Input: part model. Units: mm. Frame: model coordinates. Round coordinates to 2 decimals unless told otherwise and drop trailing zeros. Loops run counter-clockwise (first coordinate to the right, second up) from the corner with the lowest first, then second, coordinate; pieces in that order, holes last. Notation, with made-up numbers: (2, -32) -> (44, -32) arc R22 ccw to (44, -25) -> close; hole circle Ø3 at (87.25, -16.75). An arc over 180 degrees is marked (long way). Answer as a JSON object with one key per item and string values.
```python
from build123d import *

# Parameters (mm, degrees)
CYLINDER007_R     = 1.75
CYLINDER007_DEPTH = 5
CYLINDER006_R     = 1.75
CYLINDER006_DEPTH = 5
CYLINDER005_R     = 1.75
CYLINDER005_DEPTH = 5
CYLINDER004_R     = 1.75
CYLINDER004_DEPTH = 5
CUBE002_W         = 85
CUBE002_H         = 27
CUBE002_DEPTH     = 17
CYLINDER011_R     = 1.75
CYLINDER011_DEPTH = 5
CYLINDER010_R     = 1.75
CYLINDER010_DEPTH = 5
CYLINDER009_R     = 1.75
CYLINDER009_DEPTH = 5
CYLINDER008_R     = 1.75
CYLINDER008_DEPTH = 5
CUBE003_W         = 95.25
CUBE003_H         = 50.8
CUBE003_DEPTH     = 20.32
CYLINDER015_R     = 1.75
CYLINDER015_DEPTH = 5
CYLINDER014_R     = 1.75
CYLINDER014_DEPTH = 5
CYLINDER013_R     = 1.75
CYLINDER013_DEPTH = 5
CYLINDER012_R     = 1.75
CYLINDER012_DEPTH = 5
CUBE004_W         = 65
CUBE004_H         = 38
CUBE004_DEPTH     = 10
CUBE005_W         = 10
CUBE005_H         = 109
CUBE005_DEPTH     = 10
CYLINDER019_R     = 1.75
CYLINDER019_DEPTH = 5
CYLINDER018_R     = 1.75
CYLINDER018_DEPTH = 5
CYLINDER017_R     = 1.75
CYLINDER017_DEPTH = 5
CYLINDER016_R     = 1.75
CYLINDER016_DEPTH = 5
CUBE006_W         = 55
CUBE006_H         = 55
CUBE006_DEPTH     = 10
CYLINDER020_R     = 10
CYLINDER020_DEPTH = 20
CYLINDER021_R     = 10
CYLINDER021_DEPTH = 20
CYLINDER003_R     = 1.75
CYLINDER003_DEPTH = 5
CYLINDER002_R     = 1.75
CYLINDER002_DEPTH = 5
CYLINDER001_R     = 1.75
CYLINDER001_DEPTH = 5
CYLINDER_R        = 1.75
CYLINDER_DEPTH    = 5
CUBE001_W         = 45
CUBE001_H         = 25
CUBE001_DEPTH     = 12
CUBE_W            = 218
CUBE_H            = 129
CUBE_DEPTH        = 2


with BuildPart() as cylinder007:
    # cylinder007 → cylinder007 (new body)
    with BuildSketch(Plane(origin=(28, 10, -5), x_dir=(1, 0, 0), z_dir=(0, 0, 1))):
        Circle(CYLINDER007_R)
    extrude(amount=CYLINDER007_DEPTH)


with BuildPart() as group005:
    # cylinder006 → cylinder006 (new body)
    with BuildSketch(Plane(origin=(28, -10, -5), x_dir=(1, 0, 0), z_dir=(0, 0, 1))):
        Circle(CYLINDER006_R)
    extrude(amount=CYLINDER006_DEPTH)

    # Group005: union cylinder007
    add(cylinder007.part)


with BuildPart() as cylinder005:
    # cylinder005 → cylinder005 (new body)
    with BuildSketch(Plane(origin=(-28, 10, -5), x_dir=(1, 0, 0), z_dir=(0, 0, 1))):
        Circle(CYLINDER005_R)
    extrude(amount=CYLINDER005_DEPTH)


with BuildPart() as group006:
    # cylinder004 → cylinder004 (new body)
    with BuildSketch(Plane(origin=(-28, -10, -5), x_dir=(1, 0, 0), z_dir=(0, 0, 1))):
        Circle(CYLINDER004_R)
    extrude(amount=CYLINDER004_DEPTH)

    # Group004: union cylinder005
    add(cylinder005.part)

    # Group006: union Group005
    add(group005.part)


with BuildPart() as group007:
    # cube002 → cube002 (new body)
    with BuildSketch(Plane(origin=(-42.5, -13.5, 0), x_dir=(1, 0, 0), z_dir=(0, 0, 1))):
        with Locations((42.5, 13.5)):
            Rectangle(CUBE002_W, CUBE002_H)
    extrude(amount=CUBE002_DEPTH)

    # Group007: union Group006
    add(group006.part)


with BuildPart() as group007_1:
    # Group007 placement: moved
    add(group007.part.moved(Location((80, 111.5, 0.1))))


with BuildPart() as cylinder011:
    # cylinder011 → cylinder011 (new body)
    with BuildSketch(Plane(origin=(42.85, 20.625, -5), x_dir=(1, 0, 0), z_dir=(0, 0, 1))):
        Circle(CYLINDER011_R)
    extrude(amount=CYLINDER011_DEPTH)


with BuildPart() as group009:
    # cylinder010 → cylinder010 (new body)
    with BuildSketch(Plane(origin=(42.85, -20.625, -5), x_dir=(1, 0, 0), z_dir=(0, 0, 1))):
        Circle(CYLINDER010_R)
    extrude(amount=CYLINDER010_DEPTH)

    # Group009: union cylinder011
    add(cylinder011.part)


with BuildPart() as cylinder009:
    # cylinder009 → cylinder009 (new body)
    with BuildSketch(Plane(origin=(-42.85, 20.625, -5), x_dir=(1, 0, 0), z_dir=(0, 0, 1))):
        Circle(CYLINDER009_R)
    extrude(amount=CYLINDER009_DEPTH)


with BuildPart() as group010:
    # cylinder008 → cylinder008 (new body)
    with BuildSketch(Plane(origin=(-42.85, -20.625, -5), x_dir=(1, 0, 0), z_dir=(0, 0, 1))):
        Circle(CYLINDER008_R)
    extrude(amount=CYLINDER008_DEPTH)

    # Group008: union cylinder009
    add(cylinder009.part)

    # Group010: union Group009
    add(group009.part)


with BuildPart() as group011:
    # cube003 → cube003 (new body)
    with BuildSketch(Plane(origin=(-47.625, -25.4, 0), x_dir=(1, 0, 0), z_dir=(0, 0, 1))):
        with Locations((47.625, 25.4)):
            Rectangle(CUBE003_W, CUBE003_H)
    extrude(amount=CUBE003_DEPTH)

    # Group011: union Group010
    add(group010.part)


with BuildPart() as group011_1:
    # Group011 placement: moved
    add(group011.part.moved(Location((67.625, 70, 0.1))))


with BuildPart() as cylinder015:
    # cylinder015 → cylinder015 (new body)
    with BuildSketch(Plane(origin=(29, 16, -5), x_dir=(1, 0, 0), z_dir=(0, 0, 1))):
        Circle(CYLINDER015_R)
    extrude(amount=CYLINDER015_DEPTH)


with BuildPart() as group013:
    # cylinder014 → cylinder014 (new body)
    with BuildSketch(Plane(origin=(29, -16, -5), x_dir=(1, 0, 0), z_dir=(0, 0, 1))):
        Circle(CYLINDER014_R)
    extrude(amount=CYLINDER014_DEPTH)

    # Group013: union cylinder015
    add(cylinder015.part)


with BuildPart() as cylinder013:
    # cylinder013 → cylinder013 (new body)
    with BuildSketch(Plane(origin=(-29, 16, -5), x_dir=(1, 0, 0), z_dir=(0, 0, 1))):
        Circle(CYLINDER013_R)
    extrude(amount=CYLINDER013_DEPTH)


with BuildPart() as group014:
    # cylinder012 → cylinder012 (new body)
    with BuildSketch(Plane(origin=(-29, -16, -5), x_dir=(1, 0, 0), z_dir=(0, 0, 1))):
        Circle(CYLINDER012_R)
    extrude(amount=CYLINDER012_DEPTH)

    # Group012: union cylinder013
    add(cylinder013.part)

    # Group014: union Group013
    add(group013.part)


with BuildPart() as group015:
    # cube004 → cube004 (new body)
    with BuildSketch(Plane(origin=(-32.5, -19, 0), x_dir=(1, 0, 0), z_dir=(0, 0, 1))):
        with Locations((32.5, 19)):
            Rectangle(CUBE004_W, CUBE004_H)
    extrude(amount=CUBE004_DEPTH)

    # Group015: union Group014
    add(group014.part)


with BuildPart() as group015_1:
    # Group015 placement: moved
    add(group015.part.moved(Location((79, 23, 0.1))))


with BuildPart() as cube005:
    # cube005 → cube005 (new body)
    with BuildSketch(Plane(origin=(0, 10, -5), x_dir=(1, 0, 0), z_dir=(0, 0, 1))):
        with Locations((5, 54.5)):
            Rectangle(CUBE005_W, CUBE005_H)
    extrude(amount=CUBE005_DEPTH)


with BuildPart() as cylinder019:
    # cylinder019 → cylinder019 (new body)
    with BuildSketch(Plane(origin=(22.5, 22.5, -5), x_dir=(1, 0, 0), z_dir=(0, 0, 1))):
        Circle(CYLINDER019_R)
    extrude(amount=CYLINDER019_DEPTH)


with BuildPart() as group017:
    # cylinder018 → cylinder018 (new body)
    with BuildSketch(Plane(origin=(22.5, -22.5, -5), x_dir=(1, 0, 0), z_dir=(0, 0, 1))):
        Circle(CYLINDER018_R)
    extrude(amount=CYLINDER018_DEPTH)

    # Group017: union cylinder019
    add(cylinder019.part)


with BuildPart() as cylinder017:
    # cylinder017 → cylinder017 (new body)
    with BuildSketch(Plane(origin=(-22.5, 22.5, -5), x_dir=(1, 0, 0), z_dir=(0, 0, 1))):
        Circle(CYLINDER017_R)
    extrude(amount=CYLINDER017_DEPTH)


with BuildPart() as group018:
    # cylinder016 → cylinder016 (new body)
    with BuildSketch(Plane(origin=(-22.5, -22.5, -5), x_dir=(1, 0, 0), z_dir=(0, 0, 1))):
        Circle(CYLINDER016_R)
    extrude(amount=CYLINDER016_DEPTH)

    # Group016: union cylinder017
    add(cylinder017.part)

    # Group018: union Group017
    add(group017.part)


with BuildPart() as group019:
    # cube006 → cube006 (new body)
    with BuildSketch(Plane(origin=(-27.5, -27.5, 0), x_dir=(1, 0, 0), z_dir=(0, 0, 1))):
        with Locations((27.5, 27.5)):
            Rectangle(CUBE006_W, CUBE006_H)
    extrude(amount=CUBE006_DEPTH)

    # Group019: union Group018
    add(group018.part)


with BuildPart() as group019_1:
    # Group019 placement: moved
    add(group019.part.moved(Location((77.5, 70, 0.1))))


with BuildPart() as cylinder020:
    # cylinder020 → cylinder020 (new body)
    with BuildSketch(Plane(origin=(160, 70, -5), x_dir=(1, 0, 0), z_dir=(0, 0, 1))):
        Circle(CYLINDER020_R)
    extrude(amount=CYLINDER020_DEPTH)


with BuildPart() as cylinder021:
    # cylinder021 → cylinder021 (new body)
    with BuildSketch(Plane(origin=(30, 70, -5), x_dir=(1, 0, 0), z_dir=(0, 0, 1))):
        Circle(CYLINDER021_R)
    extrude(amount=CYLINDER021_DEPTH)


with BuildPart() as cylinder003:
    # cylinder003 → cylinder003 (new body)
    with BuildSketch(Plane(origin=(19.5, 9.5, -5), x_dir=(1, 0, 0), z_dir=(0, 0, 1))):
        Circle(CYLINDER003_R)
    extrude(amount=CYLINDER003_DEPTH)


with BuildPart() as group001:
    # cylinder002 → cylinder002 (new body)
    with BuildSketch(Plane(origin=(19.5, -9.5, -5), x_dir=(1, 0, 0), z_dir=(0, 0, 1))):
        Circle(CYLINDER002_R)
    extrude(amount=CYLINDER002_DEPTH)

    # Group001: union cylinder003
    add(cylinder003.part)


with BuildPart() as cylinder001:
    # cylinder001 → cylinder001 (new body)
    with BuildSketch(Plane(origin=(-19.5, 9.5, -5), x_dir=(1, 0, 0), z_dir=(0, 0, 1))):
        Circle(CYLINDER001_R)
    extrude(amount=CYLINDER001_DEPTH)


with BuildPart() as group002:
    # cylinder → cylinder (new body)
    with BuildSketch(Plane(origin=(-19.5, -9.5, -5), x_dir=(1, 0, 0), z_dir=(0, 0, 1))):
        Circle(CYLINDER_R)
    extrude(amount=CYLINDER_DEPTH)

    # Group: union cylinder001
    add(cylinder001.part)

    # Group002: union Group001
    add(group001.part)


with BuildPart() as union:
    # cube001 → cube001 (new body)
    with BuildSketch(Plane(origin=(-22.5, -12.5, 0), x_dir=(1, 0, 0), z_dir=(0, 0, 1))):
        with Locations((22.5, 12.5)):
            Rectangle(CUBE001_W, CUBE001_H)
    extrude(amount=CUBE001_DEPTH)

    # Group003: union Group002
    add(group002.part)


with BuildPart() as union_1:
    # Group003 placement: moved
    add(union.part.moved(Location((193.5, 111.5, 0.1))))

    # union: union Group007, Group011, Group015, cube005, Group019, cylinder020, cylinder021
    add(group007_1.part)
    add(group011_1.part)
    add(group015_1.part)
    add(cube005.part)
    add(group019_1.part)
    add(cylinder020.part)
    add(cylinder021.part)


with BuildPart() as difference:
    # cube → cube (new body)
    with BuildSketch(Plane.XY.offset(-2)):
        with Locations((109, 64.5)):
            Rectangle(CUBE_W, CUBE_H)
    extrude(amount=CUBE_DEPTH)

    # difference: cut union
    add(union_1.part, mode=Mode.SUBTRACT)


solid = difference.part
```
1) Section B-B, the plane x = 158. Output: boundary loops of the cut face in (y, z), plus the area to 3 significant figures.
Output:
{"outline": "(0, -2) -> (60.2, -2) -> (60.2, 0) -> (0, 0) -> close; (79.8, -2) -> (129, -2) -> (129, 0) -> (79.8, 0) -> close", "area": "219 mm^2"}
2) Contact query for flat-ended pins moving along their axis: P1, Ø3, axis at x = 108, y = 39, coming from the +Z side (3 decimals); P2, Ø1, axis at y = 38, z = -1, coming from the -X side. Output: stop coordinate, or through.
Output:
{"P1": "passes through", "P2": "stops at x = 10"}
3) Ray query, probe 1 along X at (y, z) = (47.5, -1.4); probe 2 along X at (y, z) = (70, -0.35); probe 3 along Y at (x, z) = (50, -0.9). Return the intervals inside material, ascending.
Output:
{"probe 1": "x = 10 to 53.25, 56.75 to 98.25, 101.75 to 218", "probe 2": "x = 10 to 20, 40 to 150, 170 to 218", "probe 3": "y = 0 to 5.25, 8.75 to 37.25, 40.75 to 129"}
4) Section C-C, the plane z = -1.6. Count the separate pieces of the cut face and the enclosed holes in it, plus the area to 3 significant figures.
Output:
{"separate pieces": "1", "enclosed holes": "22", "area": "26,200 mm^2"}
5) Section A-A, the plane y = 70. Output: boundary loops of the cut face in (x, z).
Output:
{"outline": "(10, -2) -> (20, -2) -> (20, 0) -> (10, 0) -> close; (40, -2) -> (150, -2) -> (150, 0) -> (40, 0) -> close; (170, -2) -> (218, -2) -> (218, 0) -> (170, 0) -> close"}
6) Draft query along Y for faces 1 (the face through (169.54, 73, -1.01)), 2 (the face through (107, 65, 0)). Return one class per face: +Y half, -Y half, draft (parallel to the pull), parting line (faces both ways), or undercut.
Output:
{"face 1": "undercut", "face 2": "draft"}
7) Section D-D, the plane y = 31.5. Output: boundary loops of the cut face in (x, z), plus the area to 3 significant figures.
Output:
{"outline": "(10, -2) -> (218, -2) -> (218, 0) -> (10, 0) -> close", "area": "416 mm^2"}
